Autodesk Inventor part; units mm, degrees
ref_plane "YZ Plane" through (0, 0, 0) normal (1, 0, 0) x (0, 1, 0)
ref_plane "XZ Plane" through (0, 0, 0) normal (0, 1, 0) x (-1, 0, 0)
ref_plane "XY Plane" through (0, 0, 0) normal (0, 0, 1) x (1, 0, 0)
sketch "Sketch1" plane through (0, 0, 0) normal (0, 1, 0) x (-1, 0, 0)
  line L0 (-11.1125, 25.4) -> (11.1125, 25.4)
  line L1 (11.1125, 25.4) -> (11.1125, -25.4)
  line L2 (11.1125, -25.4) -> (-11.1125, -25.4)
  line L3 (-11.1125, -25.4) -> (-11.1125, 25.4)
  line L4 (-11.1125, 25.4) -> (11.1125, -25.4) construction
  line L5 (11.1125, 25.4) -> (-11.1125, -25.4) construction
  point P0 (0, 0)
  dimension "d0" = 22.225
  dimension "d1" = 50.8
extrude "Extrusion1" add sketch "Sketch1" along normal blind 5.842
sketch "Sketch2" plane through (0, 5.842, 0) normal (0, 1, 0) x (1, 0, 0)
  line L0 (-11.1125, -25.4) -> (11.1125, -25.4) construction
  line L1 (0, -25.4) -> (0, 25.4) construction
  line L2 (11.1125, 25.4) -> (-11.1125, 25.4) construction
  line L3 (-11.1125, 25.4) -> (-11.1125, -25.4) construction
  line L4 (-11.1125, 0) -> (11.1125, 0) construction
  line L5 (11.1125, -25.4) -> (11.1125, 25.4) construction
  line L6 (6.35, 0) -> (-6.35, 0) construction
  line L7 (6.35, 1.5875) -> (-6.35, 1.5875)
  line L8 (-6.35, -1.5875) -> (6.35, -1.5875)
  arc A0 (6.35, -1.5875) -> (6.35, 1.5875) centre (6.35, 0) ccw
  arc A1 (-6.35, 1.5875) -> (-6.35, -1.5875) centre (-6.35, 0) ccw
  line L9 (0, -6.35) -> (0, 6.35) construction
  line L10 (1.5875, -6.35) -> (1.5875, 6.35)
  line L11 (-1.5875, 6.35) -> (-1.5875, -6.35)
  arc A2 (-1.5875, -6.35) -> (1.5875, -6.35) centre (0, -6.35) ccw
  arc A3 (1.5875, 6.35) -> (-1.5875, 6.35) centre (0, 6.35) ccw
  line L12 (6.35, -22.225) -> (-6.35, -22.225)
  line L13 (-6.35, -22.225) -> (-6.35, -9.525)
  line L14 (-6.35, -9.525) -> (6.35, -9.525)
  line L15 (6.35, -9.525) -> (6.35, -22.225)
  line L16 (6.35, -22.225) -> (-6.35, -9.525) construction
  line L17 (-6.35, -22.225) -> (6.35, -9.525) construction
  line L18 (6.35, 22.225) -> (-6.35, 22.225)
  line L19 (-6.35, 22.225) -> (-6.35, 9.525)
  line L20 (-6.35, 9.525) -> (6.35, 9.525)
  line L21 (6.35, 9.525) -> (6.35, 22.225)
  line L22 (6.35, 22.225) -> (-6.35, 9.525) construction
  line L23 (-6.35, 22.225) -> (6.35, 9.525) construction
  line L24 (6.35, -6.35) -> (-6.35, -6.35) construction
  line L25 (-6.35, -6.35) -> (-6.35, 6.35) construction
  line L26 (-6.35, 6.35) -> (6.35, 6.35) construction
  line L27 (6.35, 6.35) -> (6.35, -6.35) construction
  line L28 (6.35, -6.35) -> (-6.35, 6.35) construction
  line L29 (-6.35, -6.35) -> (6.35, 6.35) construction
  circle A4 centre (-6.35, -6.35) radius 1.7526
  circle A5 centre (-6.35, 6.35) radius 1.7526
  circle A6 centre (6.35, -6.35) radius 1.7526
  circle A7 centre (6.35, 6.35) radius 1.7526
  point P0 (0, 0)
  point P1 (0, -15.875)
  point P2 (0, 15.875)
  point P3 (-1.5875, 1.5875)
  point P4 (-1.5875, -1.5875)
  point P5 (1.5875, -1.5875)
  point P6 (1.5875, 1.5875)
  dimension "d4" = 6.35
  dimension "d5" = 3.175
  dimension "d6" = 6.35
  dimension "d7" = 3.175
  dimension "d8" = 12.7
  dimension "d9" = 12.7
  dimension "d10" = 9.525
  dimension "d11" = 12.7
  dimension "d12" = 12.7
  dimension "d13" = 3.5052
  dimension "d14" = 3.5052
  dimension "d15" = 3.5052
  dimension "d16" = 3.5052
extrude "Extrusion2" cut sketch "Sketch2" against normal blind 4.7625
fillet "Fillet1" radius 1.5875 8 edges at (-6.35, 3.4608, 22.225) (-6.35, 3.4608, 9.525) (6.35, 3.4608, 22.225) (6.35, 3.4608, 9.525) (-6.35, 3.4608, -9.525) (-6.35, 3.4608, -22.225) (6.35, 3.4608, -22.225) (6.35, 3.4608, -9.525)
chamfer "Chamfer1" distance 1.5875 angle 45 2 edges at (4.5974, 5.842, 6.35) (-8.1026, 5.842, -6.35)
chamfer "Chamfer2" distance 0.3969 angle 45 12 edges at (-1.5875, 5.842, -3.9687) (0, 5.842, -7.9375) (1.5875, 5.842, -3.9687) (-3.9688, 5.842, -1.5875) (-7.9375, 5.842, 0) (-3.9687, 5.842, 1.5875) (-1.5875, 5.842, 3.9687) (0, 5.842, 7.9375) (1.5875, 5.842, 3.9687) (3.9687, 5.842, -1.5875) (7.9375, 5.842, 0) (3.9688, 5.842, 1.5875)
fillet "Fillet2" radius 1.5875 8 edges at (-5.885, 1.0795, 21.76) (-6.35, 1.0795, 15.875) (-5.885, 1.0795, 9.99) (0, 1.0795, 9.525) (5.885, 1.0795, 9.99) (6.35, 1.0795, 15.875) (5.885, 1.0795, 21.76) (0, 1.0795, 22.225)
properties part number "Recipe Test A"
Could you check a few things on this model? Use its own coordinates, in mm. Give positions to 0.01 mm unless a question says otherwise; leave off trailing zeros. Order: outer loops, then holes, each group sorted by start corner. A loop starts at its lowest first (then second) coordinate and runs counter-clockwise, first axis right, second up.
Q1. Suppose I cut it at B-B, the plane z = 0. Write out the boundary of the cut face in (x, y), and give its area (3 significant figures).
Q2. Suppose I cut it at D-D, the plane z = -12.5. Write out the boundary of the cut face in (x, y), and give its area (3 significant figures).
Q3. Suppose I cut it at A-A, the plane x = 0. Write out the boundary of the cut face in (y, z) (1 decimal).
Q4. Suppose I cut it at C-C, the plane y = 3.2. Count the separate pieces of the cut face and the enclosed holes in it, and give its area (3 significant figures).
Q5. If I drill on line 1 along Z through (x, y) = (-4.5, 3.75) (1 decimal); line 2 along Z through (x, y) = (0, 3.65) (1 decimal); line 3 along X through (y, z) = (2.35, 6.35), over which ranges is the centre line in solid material (lowest first)?
Q6. We'd pull the mould along X, two halves only. Please class faces 1 (the flat face through (2.6, 5.842, 6)), 2 (the flat face through (11.112, 3, 0)), 3 (the flat face through (-1.588, 3, 4)): +X half, -X half, draft (parallel to the pull), parting line (faces both ways), or undercut.
Q7. I'm going to push flat-ended pins straight in: P1, Ø10.5, axis at x = 0, z = 16.5, coming from the +Y side; P2, Ø1.5, axis at x = -0.5, z = -6, coming from the +Y side. Where does each tip first touch, or does it pass through?
Solution:
1. outline: (-11.11, 0) - (11.11, 0) - (11.11, 5.84) - (8.33, 5.84) - (7.94, 5.45) - (7.94, 1.08) - (-7.94, 1.08) - (-7.94, 5.45) - (-8.33, 5.84) - (-11.11, 5.84) - close
1. area: 54.1 mm2
2. outline: (-11.11, 0) - (11.11, 0) - (11.11, 5.84) - (6.35, 5.84) - (6.35, 1.08) - (-6.35, 1.08) - (-6.35, 5.84) - (-11.11, 5.84) - close
2. area: 69.4 mm2
3. outline: (0, -25.4) - (5.8, -25.4) - (5.8, -22.2) - (1.1, -22.2) - (1.1, -9.5) - (5.8, -9.5) - (5.8, -8.3) - (5.4, -7.9) - (1.1, -7.9) - (1.1, 7.9) - (5.4, 7.9) - (5.8, 8.3) - (5.8, 9.5) - (2.7, 9.5) arc R1.6 cw to (1.1, 11.1) - (1.1, 20.6) arc R1.6 cw to (2.7, 22.2) - (5.8, 22.2) - (5.8, 25.4) - (0, 25.4) - close
4. separate pieces: 1
4. enclosed holes: 7
4. area: 686 mm2
5. line 1: z = -25.4 to -22.2, -9.5 to -1.6, 1.6 to 9.5, 22.2 to 25.4
5. line 2: z = -25.4 to -22.2, -9.5 to -7.9, 7.9 to 9.5, 22.2 to 25.4
5. line 3: x = -11.11 to -8.1, -4.6 to -1.59, 1.59 to 4.6, 8.1 to 11.11
6. face 1: draft
6. face 2: +X half
6. face 3: undercut
7. P1: stops at y = 1.53
7. P2: stops at y = 1.08
